Design review of the part built by this model. Coordinates are the model's own, in mm. A direction names the side the tool comes from. Give positions to 0.01 mm unless a question says otherwise; leave off trailing zeros. Order: outer loops, then holes, each group sorted by start corner. A loop starts at its lowest first (then second) coordinate and runs counter-clockwise, first axis right, second up.
```python
from build123d import *

# Parameters (mm, degrees)
SKETCH1_R           = 46.875
BOSS_EXTRUDE1_DEPTH = 100
BOSS_EXTRUDE2_DEPTH = 30
SKETCH3_W           = 34.75208614
SKETCH3_H           = 130
CUT_EXTRUDE1_DEPTH  = 20


with BuildPart() as part:
    # Sketch1 → Boss-Extrude1 (new body)
    with BuildSketch(Plane.XY):
        Circle(SKETCH1_R)
    extrude(amount=BOSS_EXTRUDE1_DEPTH)

    # Sketch2 → Boss-Extrude2 (add)
    with BuildSketch(Plane.XY.offset(100)):
        Polygon((92.37604307, 0), (46.188021535, 80), (-46.188021535, 80), (-92.37604307, 0), (-46.188021535, -80), (46.188021535, -80), align=None)
    extrude(amount=BOSS_EXTRUDE2_DEPTH)

    # Sketch3 → Cut-Extrude1 (cut)
    with BuildSketch(Plane.XY.offset(130)):
        Rectangle(SKETCH3_W, SKETCH3_H)
    extrude(amount=-CUT_EXTRUDE1_DEPTH, mode=Mode.SUBTRACT)


solid = part.part
```
1. Take a section at C-C (z = 70). State the section outline as (x, y) points (3 decimals).
Recorded:
outline: circle Ø93.75 at (0, 0)
2. Draft analysis for pull direction X (two halves, no side actions). For faces 3 (the face through (-17.376, -1, 120)), 4 (the face through (25.2, 39.525, 49.3)), 5 (the face through (40, 37, 100)), state which applies: pulls with the +X half, pulls with the -X half, needs draft (parallel to the pull), parting line crosses it, or undercut.
Recorded:
face 3: undercut
face 4: parting line crosses it
face 5: needs draft
3. Machinability: for faces 1 (the face through (-1, -80, 115)), 2 (the face through (0, 65, 120)), which of the approach directions +Z, -Z, +X, -X, +Y, -Y give a long, thin tool a straight path to every point of the face, cutting with its end or side? Answer none if there is none.
Recorded:
face 1: +Z, -Z, +X, -X, -Y
face 2: +Z
4. For pin 1 (1.5 mm diameter, centred on x = 4, z = 29, fed in from +Y); pin 2 (16 mm diameter, centred on y = -10, z = 121, fed in from +X); pin 3 (10 mm diameter, centred on x = 14.5, z = 28, fed in from +Y), all flat-tipped, find the tip position at first contact; note any pin that passes through.
Recorded:
pin 1: stops at y = 46.76
pin 2: stops at x = 91.22
pin 3: stops at y = 45.9
5. Take a section at D-D (x = 30.5). State the section outline as (y, z) points, then the cut area to 3 significant figures.
Recorded:
outline: (-80, 100) - (-35.6, 100) - (-35.6, 0) - (35.6, 0) - (35.6, 100) - (80, 100) - (80, 130) - (-80, 130) - close
area: 11,900 mm2
6. Take a section at A-A (x = 0). State the section outline as (y, z) points (3 decimals).
Recorded:
outline: (-80, 100) - (-46.875, 100) - (-46.875, 0) - (46.875, 0) - (46.875, 100) - (80, 100) - (80, 130) - (65, 130) - (65, 110) - (-65, 110) - (-65, 130) - (-80, 130) - close
7. Take a section at B-B (y = 9). State the section outline as (x, z) points, then the cut area to 3 significant figures.
Recorded:
outline: (-87.18, 100) - (-46, 100) - (-46, 0) - (46, 0) - (46, 100) - (87.18, 100) - (87.18, 130) - (17.38, 130) - (17.38, 110) - (-17.38, 110) - (-17.38, 130) - (-87.18, 130) - close
area: 13,700 mm2
8. For line 1 along Y through (x, z) = (-2, 9.5); line 2 along Z through (x, y) = (-70, 32.5); line 3 along X through (y, z) = (56, 124.5), list the stretches that pass through material, from the lowest coordinate up.
Recorded:
line 1: y = -46.83 to 46.83
line 2: z = 100 to 130
line 3: x = -60.04 to -17.38, 17.38 to 60.04
